Autodesk Inventor part; units mm, degrees
ref_plane "YZ Plane" through (0, 0, 0) normal (1, 0, 0) x (0, 1, 0)
ref_plane "XZ Plane" through (0, 0, 0) normal (0, 1, 0) x (-1, 0, 0)
ref_plane "XY Plane" through (0, 0, 0) normal (0, 0, 1) x (1, 0, 0)
sketch "Skizze1" plane through (0, 0, 0) normal (0, 1, 0) x (-1, 0, 0)
  line L0 (-4.6, 12.6) -> (-4.6, 0)
  arc A0 (-4.6, 0) -> (0, -4.6) centre (0, 0) ccw
  line L1 (0, -4.6) -> (12.6, -4.6)
  arc A1 (12.6, -4.6) -> (17.2, 0) centre (12.6, 0) ccw
  line L2 (17.2, 0) -> (0, 0)
  line L3 (0, 0) -> (0, 17.2)
  arc A2 (0, 17.2) -> (-4.6, 12.6) centre (0, 12.6) ccw
  point P0 (0, 0)
  dimension "d0" = 4.6
  dimension "d1" = 21.8
extrude "Extrusion1" add sketch "Skizze1" along normal blind 227.2
sketch "Skizze2" plane through (0, 0, -4.6) normal (0, 0, -1) x (-1, 0, 0)
  line L0 (-4.6, 0) -> (17.2, 21.8)
  line L1 (17.2, 0) -> (17.2, 227.2)
  line L2 (17.2, 0) -> (12.6, 0)
  line L3 (17.2, 21.8) -> (17.2, 0)
  line L4 (17.2, 0) -> (-4.6, 0)
  line L5 (17.2, 227.2) -> (-4.6, 227.2)
  line L6 (-4.6, 227.2) -> (17.2, 205.4)
  line L7 (17.2, 227.2) -> (17.2, 205.4)
  point P0 (0, 0)
  dimension "d4" = 45
  dimension "d7" = 45
extrude "Extrusion2" cut sketch "Skizze2" against normal through all
sketch "Skizze3" plane through (4.6, 0, 0) normal (1, 0, 0) x (0, 0, -1)
  line L0 (4.6, 0) -> (-17.2, 21.8)
  line L1 (-17.2, 4.6) -> (-17.2, 222.6)
  line L2 (-17.2, 21.8) -> (-17.2, 0)
  line L3 (-17.2, 0) -> (4.6, 0)
  line L4 (-17.2, 205.4) -> (-17.2, 227.2)
  line L5 (-17.2, 227.2) -> (4.6, 227.2)
  line L6 (4.6, 227.2) -> (-17.2, 205.4)
  point P0 (0, 0)
  point P1 (4.6, 4.6)
  point P2 (-12.6, 227.2)
  dimension "d8" = 45
  dimension "d9" = 45
extrude "Extrusion3" cut sketch "Skizze3" against normal through all
properties part number "winkelTop" material "Kiefer"
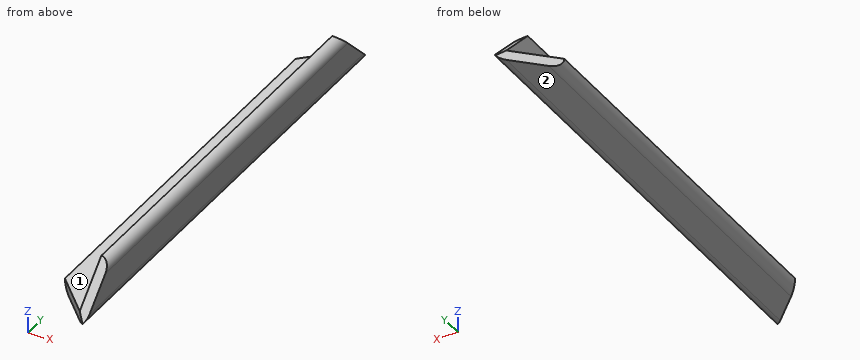
Input: part model. Units: mm. Frame: model coordinates. Face numbers are marked on the shaded views. A direction names the side the tool comes from. Give positions to 0.01 mm unless a question says otherwise; leave off trailing zeros. Order: outer loops, then holes, each group sorted by start corner. A loop starts at its lowest first (then second) coordinate and runs counter-clockwise, first axis right, second up. Notation, with made-up numbers: M 32.5,-31 L 39.5,-31 A21 ccw 39.5,-19 Z; hole C 2,54 d3. An arc over 180 degrees is marked long. Return JSON: item names as keys, results as strings.
Item 1: Ray query, probe 1 along X at (y, z) = (130.5, 5.75); probe 2 along Z at (x, y) = (-12.25, 28); probe 3 along Y at (x, z) = (-3, -2). Return the intervals inside material, ascending.
Solutions:
{"probe 1": "0 to 4.6", "probe 2": "-4.6 to 0", "probe 3": "7.6 to 219.6"}
Item 2: Cut plane A-A (y = 183.5). Return loops of the section in (x, z).
Solutions:
{"outline": "M -17.2,0 A4.6 ccw -12.6,-4.6 L 0,-4.6 A4.6 ccw 4.6,0 L 4.6,12.6 A4.6 ccw 0,17.2 L 0,0 Z"}
Item 3: First-contact query: P1, Ø5, axis at x = -1, z = 0, coming from the +Y side; P2, Ø8, axis at x = 0, z = 4.5, coming from the +Y side; P3, Ø5, axis at x = -8, y = 127, coming from the +Z side. Flat tips, straight axial feed; report the tip coordinate or a pass-through.
Solutions:
{"P1": "y = 223.8", "P2": "y = 222.1", "P3": "z = 0"}
Item 4: Cut plane B-B (z = 8.5). Return loops of the section in (x, y), then the cut area to 3 significant figures.
Solutions:
{"outline": "M 0,13.1 L 4.6,13.1 L 4.6,214.1 L 0,214.1 Z", "area": "925 mm^2"}
Item 5: Cut plane C-C (x = -6.5). Return loops of the section in (y, z).
Solutions:
{"outline": "M 11.1,-4.6 L 216.1,-4.6 L 216.1,0 L 11.1,0 Z"}
Item 6: Access query for the marked faces 1 and 2. Directions: +Z, -Z, +X, -X, +Y, -Y. A direction counts if a zero-diameter tool reaches every point of the face in a straight line with its end or side. Return the directions, or none.
Solutions:
{"face 1": "+Z, -X, +Y, -Y", "face 2": "-Z, +X, -X, +Y, -Y"}
